```python
from build123d import *

# Parameters (mm, degrees)
SKETCH1_W          = 76.2
SKETCH1_H          = 19.0246
CUT_EXTRUDE2_START = -38.1
SKETCH2_W          = 26.9748
SKETCH2_H          = 266.7
CUT_EXTRUDE2_DEPTH = 19.05


with BuildPart() as part:
    # Sketch1 → Revolve1 (revolve)
    with BuildSketch(Plane(origin=(0, 0, 0), x_dir=(0, 1, 0), z_dir=(0, 0, 1)), mode=Mode.PRIVATE) as revolve1_sk:
        with Locations((0, 123.8377)):
            Rectangle(SKETCH1_W, SKETCH1_H)
    revolve(revolve1_sk.sketch.rotate(Axis((0, -63.5, 0), (0, 1, 0)), 270), axis=Axis((0, -63.5, 0), (0, 1, 0)))

    # Sketch2 → Cut-Extrude2 (cut)
    with BuildSketch(Plane(origin=(0, 0, 0), x_dir=(-1, 0, 0), z_dir=(0, 1, 0)).offset(CUT_EXTRUDE2_START)):
        with Locations((0, 133.35)):
            Rectangle(SKETCH2_W, SKETCH2_H)
    extrude(amount=CUT_EXTRUDE2_DEPTH, mode=Mode.SUBTRACT)


solid = part.part
```
Geometry check sheet. Reference: the model listing, model coordinates, mm. A direction names the side the tool comes from. Give positions to 0.01 mm unless a question says otherwise; leave off trailing zeros. Order: outer loops, then holes, each group sorted by start corner. A loop starts at its lowest first (then second) coordinate and runs counter-clockwise, first axis right, second up.
1. Section check D-D, the plane y = -30.5. Enter the section's corners in (x, z), and give its area (3 significant figures).
2. Section check C-C, the plane y = 10. Enter the section's corners in (x, z).
3. Gauge pin test, flat ends, axial feed: pin 1 Ø12 at (x, y) = (28, -2.5) entering from -Z; pin 2 Ø1.5 at (x, y) = (67.5, -4) entering from +Z; pin 3 Ø22 at (x, z) = (1, 123) entering from -Y. Record the tip position at first contact, or that the pin passes through.
4. Thickness scan on L1, parallel to X at y = -2, z = 0; L2, parallel to Z at x = 34.5, y = -16; L3, parallel to X at y = -7, z = 77. Record the ranges inside material, lowest first.
5. Release check for a two-part mould opening along X. For faces 3 (the face through (13.487, -29, 123)), 4 (the face through (-40.055, 0.533, -127.192)), 5 (the face through (-99, -38.1, -60)), 6 (the face through (-13.487, -29, 123)) record: pulls with the +X half, pulls with the -X half, needs draft (parallel to the pull), parting line crosses it, or undercut.
6. Section check A-A, the plane z = 0. Enter the section's corners in (x, y), and give its area (3 significant figures).
7. Access from +Z, -Z, +X, -X, +Y, -Y to the whole of each face (thin tool, end or side, straight path). Record for faces 1 (the face through (0, -19.05, 124)), 2 (the face through (-60, 38.1, 98)).
8. Section check B-B, the plane x = 0. Enter the section's corners in (y, z), and give its area (3 significant figures).
Values follow:
1. outline: (-13.49, 113.53) - (-13.49, 132.67) arc R133.35 ccw (long way) to (13.49, 132.67) - (13.49, 113.53) arc R114.33 cw (long way) to start
1. area: 14,300 mm2
2. outline: circle Ø266.7 at (0, 0); hole circle Ø228.65 at (0, 0)
3. pin 1: stops at z = -131.52
3. pin 2: stops at z = 115.44
3. pin 3: stops at y = -19.05
4. L1: x = -133.35 to -114.33, 114.33 to 133.35
4. L2: z = -128.81 to -109, 109 to 128.81
4. L3: x = -108.87 to -84.51, 84.51 to 108.87
5. face 3: undercut
5. face 4: parting line crosses it
5. face 5: needs draft
5. face 6: undercut
6. outline: (-133.35, -38.1) - (-114.33, -38.1) - (-114.33, 38.1) - (-133.35, 38.1) - close; (114.33, -38.1) - (133.35, -38.1) - (133.35, 38.1) - (114.33, 38.1) - close
6. area: 2,900 mm2
7. face 1: +Z, -Y
7. face 2: +Z, -Z, +X, -X, +Y
8. outline: (-38.1, -133.35) - (38.1, -133.35) - (38.1, -114.33) - (-38.1, -114.33) - close; (-19.05, 114.33) - (38.1, 114.33) - (38.1, 133.35) - (-19.05, 133.35) - close
8. area: 2,540 mm2
